from build123d import *

# Parameters (mm, degrees)
SKETCH1_W           = 71.7
SKETCH1_H           = 56.7
SKETCH1_W_2         = 68.5
SKETCH1_H_2         = 53.5
BOSS_EXTRUDE1_DEPTH = 32
SKETCH2_W           = 15
SKETCH2_H           = 3
BOSS_EXTRUDE2_DEPTH = 70
SKETCH3_W           = 12.3
SKETCH3_H           = 12
SKETCH3_W_2         = 9.3
SKETCH3_H_2         = 11
CUT_EXTRUDE1_DEPTH  = 1.6
SKETCH3_2_W         = 12.3
SKETCH3_2_H         = 12
SKETCH3_2_W_2       = 9.3
SKETCH3_2_H_2       = 11
CUT_EXTRUDE2_DEPTH  = 18
BOSS_EXTRUDE3_DEPTH = 3
SKETCH5_W           = 55.1
SKETCH5_H           = 1
CUT_EXTRUDE3_DEPTH  = 69.3


with BuildPart() as part:
    # Sketch1 → Boss-Extrude1 (new body)
    with BuildSketch(Plane(origin=(0, 0, 0), x_dir=(1, 0, 0), z_dir=(0, 1, 0))):
        with Locations((1.229030624, -8.245503616)):
            Rectangle(SKETCH1_W, SKETCH1_H)
        with Locations((1.229030624, -8.245503616)):
            Rectangle(SKETCH1_W_2, SKETCH1_H_2, mode=Mode.SUBTRACT)
    extrude(amount=BOSS_EXTRUDE1_DEPTH)

    # Sketch2 → Boss-Extrude2 (add)
    with BuildSketch(Plane(origin=(-33.020969376, 0, 0), x_dir=(0, 0, -1), z_dir=(1, 0, 0))):
        with Locations((-8.245503616, 16.5)):
            Rectangle(SKETCH2_W, SKETCH2_H)
    extrude(amount=BOSS_EXTRUDE2_DEPTH)

    # Sketch3 → Cut-Extrude1 (cut)
    with BuildSketch(Plane(origin=(-33.020969376, 0, 0), x_dir=(0, 0, -1), z_dir=(1, 0, 0))):
        with Locations((3.454496384, 10.1)):
            Rectangle(SKETCH3_W, SKETCH3_H)
        with Locations((-27.245503616, 9.6)):
            Rectangle(SKETCH3_W_2, SKETCH3_H_2)
    extrude(amount=-CUT_EXTRUDE1_DEPTH, mode=Mode.SUBTRACT)

    # Sketch3<2> → Cut-Extrude2 (cut)
    with BuildSketch(Plane(origin=(-33.020969376, 0, 0), x_dir=(0, 0, -1), z_dir=(1, 0, 0))):
        with Locations((3.454496384, 10.1)):
            Rectangle(SKETCH3_2_W, SKETCH3_2_H)
        with Locations((-27.245503616, 9.6)):
            Rectangle(SKETCH3_2_W_2, SKETCH3_2_H_2)
    extrude(amount=CUT_EXTRUDE2_DEPTH, mode=Mode.SUBTRACT)

    # Sketch4 → Boss-Extrude3 (add)
    with BuildSketch(Plane.XZ):
        Polygon((35.479030624, 36.595503616), (35.479030624, 34.995503616), (-33.020969376, 34.995503616), (-33.020969376, -18.504496384), (35.479030624, -18.504496384), (35.479030624, -20.104496384), (-34.620969376, -20.104496384), (-34.620969376, 36.595503616), align=None)
    extrude(amount=BOSS_EXTRUDE3_DEPTH)

    # Sketch5 → Cut-Extrude3 (cut)
    with BuildSketch(Plane(origin=(35.479030624, 0, 0), x_dir=(0, 0, -1), z_dir=(1, 0, 0))):
        with Locations((-8.245503616, -1.5)):
            Rectangle(SKETCH5_W, SKETCH5_H)
    extrude(amount=-CUT_EXTRUDE3_DEPTH, mode=Mode.SUBTRACT)


solid = part.part
The listing builds one solid part. Answer for the finished solid, in the listing's coordinates (mm). A direction names the side the tool comes from. Coordinates: 2 decimals unless noted, no trailing zeros. Write each loop counter-clockwise with the first axis right and the second up, starting at its lowest first coordinate (ties: lowest second). Pieces come first, ordered by that corner, then holes. Notation, with made-up numbers: (-9.5, 18.5) - (21.5, 18.5) arc R24 cw to (21.5, 31.5) - close; hole circle Ø7 at (41, 73). An arc over 180 degrees is marked (long way). Answer as CSV lines item,"result".
1. Find section D-D (y = 3). Give the vertices of the cut face in (x, z), plus the area to 3 significant figures.
Computed values:
outline,"(-34.62, -20.1) - (37.08, -20.1) - (37.08, 36.6) - (-34.62, 36.6) - close; hole (-33.02, -18.5) - (35.48, -18.5) - (35.48, 35) - (-33.02, 35) - close"
area,"401 mm²"
2. Find section A-A (z = 29.5). Give the vertices of the cut face in (x, y), plus the area to 3 significant figures.
Computed values:
outline,"(-34.62, -3) - (-33.02, -3) - (-33.02, -2) - (-33.82, -2) - (-33.82, -1) - (-33.02, -1) - (-33.02, 4.1) - (-34.62, 4.1) - close; (-34.62, 15.1) - (-33.02, 15.1) - (-33.02, 32) - (-34.62, 32) - close; (35.48, 0) - (37.08, 0) - (37.08, 32) - (35.48, 32) - close"
area,"88.8 mm²"
3. Find section B-B (x = -24). Give the vertices of the cut face in (y, z).
Computed values:
outline,"(-3, -20.1) - (32, -20.1) - (32, -18.5) - (-1, -18.5) - (-1, -19.3) - (-2, -19.3) - (-2, -18.5) - (-3, -18.5) - close; (-3, 35) - (-2, 35) - (-2, 35.8) - (-1, 35.8) - (-1, 35) - (32, 35) - (32, 36.6) - (-3, 36.6) - close; (15, 2.7) - (16.1, 2.7) - (16.1, 0.75) - (18, 0.75) - (18, 15.75) - (15, 15.75) - close"
4. Determine the mould class of faces 1 (the flat face through (1, 15, 8)), 2 (the flat face through (35.479, -1, 36)), 3 (the flat face through (-34, 4.1, 27)) for opening direction X: +X half, -X half, draft (parallel to the pull), parting line (faces both ways), or undercut.
Computed values:
face 1,"undercut"
face 2,"+X half"
face 3,"draft"
5. Find section C-C (y = 6.5). Give the vertices of the cut face in (x, z), plus the area to 3 significant figures.
Computed values:
outline,"(-34.62, -20.1) - (37.08, -20.1) - (37.08, 36.6) - (-34.62, 36.6) - (-34.62, 31.9) - (-33.02, 31.9) - (-33.02, 35) - (35.48, 35) - (35.48, -18.5) - (-33.02, -18.5) - (-33.02, -9.6) - (-34.62, -9.6) - close; (-34.62, 2.7) - (-33.02, 2.7) - (-33.02, 22.6) - (-34.62, 22.6) - close"
area,"366 mm²"
6. A tool of negligible diameter and unlimited length cuts with its end or side. For faces 4 (the flat face through (36, 0, 8)), 5 (the flat face through (1, 18, 8)), 6 (the flat face through (-29.1, 15.4, 2.696)), 7 (the flat face through (1, 16, 0.746)), from which of +Z, -Z, +X, -X, +Y, -Y can it reach the whole face along a straight path? Write none if from no direction.
Computed values:
face 4,"+Z, -Z, +X, -Y"
face 5,"+Y"
face 6,"-X"
face 7,"+Y, -Y"
7. Given P1, Ø1.8, axis at x = 36, z = 8.5, coming from the -Y side; P2, Ø2, axis at x = 0.5, z = 4.5, coming from the -Y side; P3, Ø2, axis at x = 28.5, z = 1.5, coming from the +Y side, each flat-ended and moving along its own axis, determine where each tip first touches the part or whether it passes through.
Computed values:
P1,"stops at y = 0"
P2,"stops at y = 15"
P3,"stops at y = 18"
8. Straight lines are drawn through the part: line 1 (Z direction, x = 16, y = 16); line 2 (Z direction, x = -30, y = 1.5); line 3 (X direction, y = 20.5, z = 32.5). For each, find the intervals that lie inside material, in ascending order. Write a range as [from, to].
Computed values:
line 1,"z = [-20.1, -18.5], [0.75, 15.75], [35, 36.6]"
line 2,"z = [-20.1, -18.5], [35, 36.6]"
line 3,"x = [-34.62, -33.02], [35.48, 37.08]"
